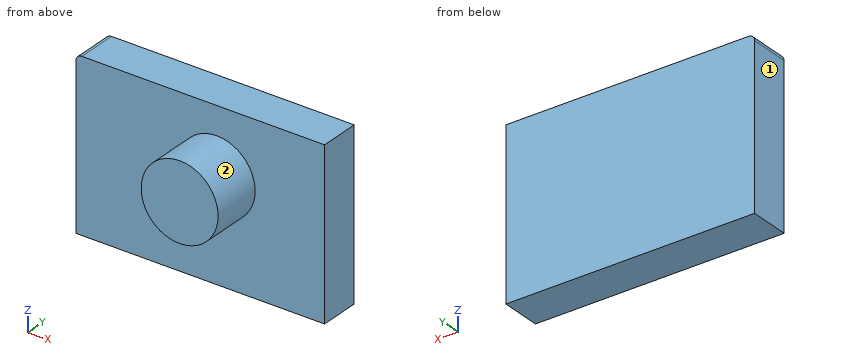
from build123d import *

# Parameters (mm, degrees)
F1_DEPTH = 20
F2_R     = 19.102377
F3_DEPTH = 25


with BuildPart() as f1:
    # F0 (on Front) → F1 (new body)
    with BuildSketch(Plane.XZ):
        with BuildLine():
            Line((53.605944, 33.028656), (-66.953859, 33.028656))
            ThreePointArc((-66.953859, 33.028656), (-69.075179, 32.149976), (-69.953859, 30.028656))
            Line((-69.953859, 30.028656), (-69.953859, -49.536757))
            Line((-69.953859, -49.536757), (53.605944, -49.536757))
            Line((53.605944, -49.536757), (53.605944, 33.028656))
        make_face()
    extrude(amount=F1_DEPTH)

    # F2 (on face) → F3 (join)
    with BuildSketch(Plane.XZ.offset(20)):
        Circle(F2_R)
    extrude(amount=F3_DEPTH)


solid = f1.part
The model under review builds one solid part; all positions refer to its coordinate system, in mm. Face numbers are marked on the shaded views. A direction names the side the tool comes from. Coordinates: 2 decimals unless noted, no trailing zeros. Loops run counter-clockwise (first coordinate to the right, second up) from the corner with the lowest first, then second, coordinate; pieces in that order, holes last. Notation, with made-up numbers: M 41,46 L 100,46 A16 cw 100,62 Z; hole C -33,-36.75 d4. An arc over 180 degrees is marked long. Put each result on its own line as item: value. Start each with the question number.
Q1. Clearance check with flat-ended pins moving along their axes: pin 1 (5 mm diameter, centred on y = -40, z = -19.5, fed in from +X); pin 2 (2 mm diameter, centred on x = 7, z = -30, fed in from -Y); pin 3 (1 mm diameter, centred on y = -21.5, z = -4.5, fed in from -X). State where each tip first meets the part, or that it passes through.
Q2. Wall thickness on line 1 (Y direction, x = 27, z = -3); line 2 (Z direction, x = -5, y = -25); line 3 (Z direction, x = -9.5, y = -24): over which ranges is each line inside the solid? List them lowest first.
Q3. Add section C-C (x = -31). Write out the cut boundary in (y, z), and give its area (3 significant figures).
Q4. Add section B-B (x = 0). Write out the cut boundary in (y, z).
Q5. Add section D-D (z = -40). Write out the cut boundary in (x, y).
Q6. Add section A-A (z = 0). Write out the cut boundary in (x, y).
Q7. For the marked faces 1 and 2, list the 3-axis set-ups (+Z, -Z, +X, -X, +Y, -Y) from which the entire face can be reached by the end or side of a thin tool; tool diameter is ignored.
Answers:
1. pin 1: stops at x = 8.71
1. pin 2: stops at y = -20
1. pin 3: stops at x = -18.68
2. line 1: y = -20 to 0
2. line 2: z = -18.44 to 18.44
2. line 3: z = -16.57 to 16.57
3. outline: M -20,-49.54 L 0,-49.54 L 0,33.03 L -20,33.03 Z
3. area: 1,650 mm^2
4. outline: M -45,-19.1 L -20,-19.1 L -20,-49.54 L 0,-49.54 L 0,33.03 L -20,33.03 L -20,19.1 L -45,19.1 Z
5. outline: M -69.95,-20 L 53.61,-20 L 53.61,0 L -69.95,0 Z
6. outline: M -69.95,-20 L -19.1,-20 L -19.1,-45 L 19.1,-45 L 19.1,-20 L 53.61,-20 L 53.61,0 L -69.95,0 Z
7. face 1: +Z, -Z, -X, +Y, -Y
7. face 2: -Y
